from build123d import *

# Parameters (mm, degrees)
F0_W     = 700
F0_H     = 1000
F1_DEPTH = 900
F2_W     = 900
F2_H     = 97.384112
F2_H_2   = 150
F2_H_3   = 650
F3_DEPTH = 1000
F4_W     = 600
F4_H     = 174.410781
F4_H_2   = 150
F4_H_3   = 650
F5_DEPTH = 1000


with BuildPart() as f1:
    # F0 (on Top) → F1 (new body)
    with BuildSketch(Plane.XY):
        Rectangle(F0_W, F0_H)
    extrude(amount=F1_DEPTH)

    # F2 (on face) → F3 (cut)
    with BuildSketch(Plane.YZ.offset(350)):
        with Locations((0, -48.692056)):
            Rectangle(F2_W, F2_H)
        with Locations((0, 75)):
            Rectangle(F2_W, F2_H_2)
        with Locations((0, 525)):
            Rectangle(F2_W, F2_H_3)
    extrude(amount=-F3_DEPTH, mode=Mode.SUBTRACT)

    # F4 (on face) → F5 (cut)
    with BuildSketch(Plane(origin=(0, 500, 0), x_dir=(-1, 0, 0), z_dir=(0, 1, 0))):
        with Locations((0, -87.20539)):
            Rectangle(F4_W, F4_H)
        with Locations((0, 75)):
            Rectangle(F4_W, F4_H_2)
        with Locations((0, 525)):
            Rectangle(F4_W, F4_H_3)
    extrude(amount=-F5_DEPTH, mode=Mode.SUBTRACT)


solid = f1.part
Verification items for the finished model (mm, model axes). A direction names the side the tool comes from. Round coordinates to 2 decimals unless told otherwise and drop trailing zeros. Loops run counter-clockwise (first coordinate to the right, second up) from the corner with the lowest first, then second, coordinate; pieces in that order, holes last. Notation, with made-up numbers: (-5, -34.75) - (45, -34.75) arc R13 ccw to (45, -9.75) - close; hole circle Ø3 at (37.25, 46). An arc over 180 degrees is marked (long way). Answer in a Markdown table with one row per item. Add a question column.
Q1. Section check B-B on y = 113. Enter the section's corners in (x, z), plus the area to 3 significant figures.
Q2. Section check C-C on x = 143. Enter the section's corners in (y, z).
Q3. Release check for a two-part mould opening along Z. For faces 1 (the face through (-300, -475, 74)), 2 (the face through (325, -450, 520)), 3 (the face through (325, 475, 0)) record: pulls with the +Z half, pulls with the -Z half, needs draft (parallel to the pull), parting line crosses it, or undercut.
Q4. Tool access check on faces 4 (the face through (-300, -475, 520)), 5 (the face through (-325, -450, 76)), 6 (the face through (325, 450, 520)). Record the directions out of +Z, -Z, +X, -X, +Y, -Y that give a thin tool (end or side, any length) a straight path to the whole face; none if there is none.
Q5. Gauge pin test, flat end, axial feed: pin 1 (10 mm diameter, centred on x = 137, y = -363.5, fed in from -Z). Record the tip position at first contact, or that the pin passes through.
Q6. Section check A-A on z = 76. Enter the section's corners in (x, y), plus the area to 3 significant figures.
Q7. Material ranges on line 1 (Z direction, x = -28, y = 12.5); line 2 (Y direction, x = -300.5, z = 729), recorded low to high.
Found:
| question | item | result |
|---|---|---|
| 1 | outline | (-350, 150) - (350, 150) - (350, 200) - (-350, 200) - close; (-350, 850) - (350, 850) - (350, 900) - (-350, 900) - close |
| 1 | area | 70,000 mm² |
| 2 | outline | (-500, 150) - (500, 150) - (500, 200) - (-500, 200) - close; (-500, 850) - (500, 850) - (500, 900) - (-500, 900) - close |
| 3 | face 1 | needs draft |
| 3 | face 2 | undercut |
| 3 | face 3 | pulls with the -Z half |
| 4 | face 4 | +Y, -Y |
| 4 | face 5 | -Z, +X, -X |
| 4 | face 6 | +X, -X |
| 5 | pin 1 | stops at z = 150 |
| 6 | outline | (-350, -500) - (-300, -500) - (-300, -450) - (-350, -450) - close; (-350, 450) - (-300, 450) - (-300, 500) - (-350, 500) - close; (300, -500) - (350, -500) - (350, -450) - (300, -450) - close; (300, 450) - (350, 450) - (350, 500) - (300, 500) - close |
| 6 | area | 10,000 mm² |
| 7 | line 1 | z = 150 to 200, 850 to 900 |
| 7 | line 2 | y = -500 to -450, 450 to 500 |
